from build123d import *

# Parameters (mm, degrees)
F0_R     = 26.5
F1_DEPTH = 15
F3_D     = 48
F5_DEPTH = 15.001


with BuildPart() as f1:
    # F0 (on Top) → F1 (new body)
    with BuildSketch(Plane.XY):
        Circle(F0_R)
    extrude(amount=F1_DEPTH)

    # F3 (through all)
    with Locations(Plane.XY.offset(15)):
        with Locations((0, 0)):
            Hole(F3_D / 2)

    # F4 (on face) → F5 (cut, through all)
    with BuildSketch(Plane.XY.offset(15)):
        with BuildLine():
            Line((26.2814522422, 3.396361), (23.7584665321, 3.396361))
            ThreePointArc((23.7584665321, 3.396361), (23.9395404798, 1.7024692698), (24, 0))
            ThreePointArc((24, 0), (23.9318812143, -1.8069481297), (23.7279115381, -3.603639))
            Line((23.727911538, -3.603639), (26.2538337383, -3.603639))
            ThreePointArc((26.2538337383, -3.603639), (26.4383868084, -1.8060185402), (26.5, 0))
            ThreePointArc((26.5, 0), (26.4453066197, 1.7016926254), (26.2814522422, 3.396361))
        make_face()
    extrude(amount=-F5_DEPTH, mode=Mode.SUBTRACT)


solid = f1.part
Design review of the part built by this model. Coordinates are the model's own, in mm. A direction names the side the tool comes from. Round coordinates to 2 decimals unless told otherwise and drop trailing zeros. Loops run counter-clockwise (first coordinate to the right, second up) from the corner with the lowest first, then second, coordinate; pieces in that order, holes last. Notation, with made-up numbers: (45.25, 0) - (87.25, 0) arc R19 cw to (87.25, 27) - close; hole circle Ø4 at (50, 85). An arc over 180 degrees is marked (long way). One line per question, with ' | ' between items.
1. For faces 1 (the face through (-20, -14, 0)), 2 (the face through (25, -3.604, 8)), list the 3-axis set-ups (+Z, -Z, +X, -X, +Y, -Y) from which the entire face can be reached by the end or side of a thin tool; tool diameter is ignored.
Results are:
face 1: -Z, +X, -X, +Y, -Y | face 2: +Z, -Z, +X
2. Draft analysis for pull direction Y (two halves, no side actions). For faces 3 (the face through (-26.47, 1.22, 7.4)), 4 (the face through (25, 3.396, 8)), 5 (the face through (-20, -14, 15)), state which applies: released by +Y, released by -Y, zero draft, split by the parting line, or undercut.
Results are:
face 3: split by the parting line | face 4: undercut | face 5: zero draft
3. We need section C-C, the plane z = 10.5. State the section outline as (x, y) points.
Results are:
outline: (23.73, -3.6) arc R24 cw (long way) to (23.76, 3.4) - (26.28, 3.4) arc R26.5 ccw (long way) to (26.25, -3.6) - close
4. We need section B-B, the plane y = 17. State the section outline as (x, z) points, and give its area (3 significant figures).
Results are:
outline: (-20.33, 0) - (-16.94, 0) - (-16.94, 15) - (-20.33, 15) - close; (16.94, 0) - (20.33, 0) - (20.33, 15) - (16.94, 15) - close | area: 102 mm²
5. Clearance check with flat-ended pins moving along their axes: P1, Ø1.5, axis at y = -4, z = 5, coming from the +X side; P2, Ø0.8, axis at x = 24.5, z = 4.5, coming from the +Y side; P3, Ø3, axis at y = -2, z = 4.5, coming from the -X side. State where each tip first meets the part, or that it passes through.
Results are:
P1: stops at x = 26.25 | P2: stops at y = 11.02 | P3: stops at x = -26.5
6. For L1, parallel to Y at x = 0, z = 9.5; L2, parallel to X at y = -20.5, z = 7.75; L3, parallel to X at y = 19.5, z = 8, list the stretches that pass through material, from the lowest coordinate up. Write a range as [from, to].
Results are:
L1: y = [-26.5, -24], [24, 26.5] | L2: x = [-16.79, -12.48], [12.48, 16.79] | L3: x = [-17.94, -13.99], [13.99, 17.94]
7. We need section A-A, the plane x = 0. State the section outline as (y, z) points.
Results are:
outline: (-26.5, 0) - (-24, 0) - (-24, 15) - (-26.5, 15) - close; (24, 0) - (26.5, 0) - (26.5, 15) - (24, 15) - close
